```python
from build123d import *

# Parameters (mm, degrees)
SKETCH_1_R      = 5
SKETCH_1_R_2    = 1.5
EXTRUDE_2_DEPTH = 3


with BuildPart() as part:
    # 草图1 → 凸台-拉伸2 (new body)
    with BuildSketch(Plane.XY):
        with BuildLine():
            ThreePointArc((0, 5), (-5, 0), (0, -5))
            add(Edge.make_bspline(
                [(0, -5), (24.095302235, -4.17152905), (70, -7)],
                knots=[0, 0, 0, 1, 1, 1], degree=2))
            ThreePointArc((70, -7), (77, 0), (70, 7))
            add(Edge.make_bspline(
                [(0, 5), (24.095302235, 4.17152905), (70, 7)],
                knots=[0, 0, 0, 1, 1, 1], degree=2))
        make_face()
        with Locations((70, 0)):
            Circle(SKETCH_1_R, mode=Mode.SUBTRACT)
        Circle(SKETCH_1_R_2, mode=Mode.SUBTRACT)
    extrude(amount=EXTRUDE_2_DEPTH)


solid = part.part
```
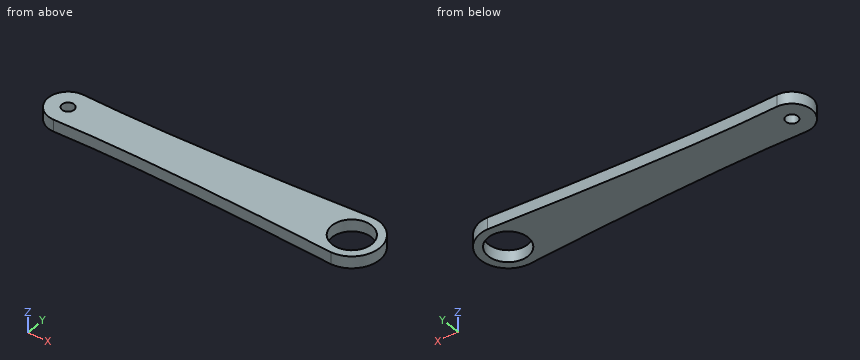
Check sheet for the modelled part. Datum: model origin and axes. Units: mm. Round coordinates to 2 decimals unless told otherwise and drop trailing zeros. Write each loop counter-clockwise with the first axis right and the second up, starting at its lowest first coordinate (ties: lowest second). Pieces come first, ordered by that corner, then holes. Notation, with made-up numbers: M 29.5,46 L 63.5,46 A20 ccw 63.5,78 Z; hole C -29,-37.75 d7. An arc over 180 degrees is marked long. Write item = value, one per line. Start each with the question number.
1. Scan lines: line 1 (Y direction, x = 0, z = 1.35); line 2 (Y direction, x = 70, z = 1.9); line 3 (Y direction, x = 14.5, z = 0.4). Record each from-to range of solid material in increasing order. Write a range as [from, to].
2. Section check A-A, the plane y = 0. Record the cut outline in (x, z), then the cut area to 3 significant figures.
3. Gauge pin test, flat end, axial feed: pin 1 (1 mm diameter, centred on y = -3, z = 2, fed in from +X). Record the tip position at first contact, or that the pin passes through.
4. Section check B-B, the plane y = -4. Record the cut outline in (x, z), then the cut area to 3 significant figures.
5. Section check C-C, the plane z = 2.1. State how many separate pieces and enclosed holes the cut face has, then the cut area to 3 significant figures.
Results found:
q1.line_1 = [-5, -1.5], [1.5, 5]
q1.line_2 = [-7, -5], [5, 7]
q1.line_3 = [-4.82, 4.82]
q2.outline = M -5,0 L -1.5,0 L -1.5,3 L -5,3 Z; M 1.5,0 L 65,0 L 65,3 L 1.5,3 Z; M 75,0 L 77,0 L 77,3 L 75,3 Z
q2.area = 207 mm^2
q3.pin_1 = 76.54
q4.outline = M -3,0 L 67,0 L 67,3 L -3,3 Z; M 73,0 L 75.74,0 L 75.74,3 L 73,3 Z
q4.area = 218 mm^2
q5.separate_pieces = 1
q5.enclosed_holes = 2
q5.area = 800 mm^2
